For this review, take the finished solid that the model builds, in its own axes (mm). Give positions to 0.01 mm unless a question says otherwise; leave off trailing zeros. Write each loop counter-clockwise with the first axis right and the second up, starting at its lowest first coordinate (ties: lowest second). Pieces come first, ordered by that corner, then holes. Notation, with made-up numbers: (18, 12) -> (74, 12) arc R19 cw to (74, 21) -> close; hole circle Ø4 at (33, 6). An arc over 180 degrees is marked (long way). Answer as CSV lines item,"result".
```python
from build123d import *

# Parameters (mm, degrees)
F1_DEPTH = 1.1557


with BuildPart() as f1:
    # F0 (on Front) → F1 (new body)
    with BuildSketch(Plane.XZ):
        with BuildLine():
            Line((0, 200), (0, 0))
            Line((0, 0), (80, 0))
            Line((80, 0), (80, 149.5))
            ThreePointArc((80, 149.5), (102.5, 172), (125, 149.5))
            Line((125, 149.5), (125, 0))
            Line((125, 0), (170, 0))
            Line((170, 0), (170, 149.5))
            ThreePointArc((170, 149.5), (192.5, 172), (215, 149.5))
            Line((215, 149.5), (215, 0))
            Line((215, 0), (318, 0))
            Line((318, 0), (318, 149.5))
            ThreePointArc((318, 149.5), (340.5, 172), (363, 149.5))
            Line((363, 149.5), (363, 0))
            Line((363, 0), (600, 0))
            Line((600, 0), (600, 200))
            Line((600, 200), (0, 200))
        make_face()
    extrude(amount=F1_DEPTH)


solid = f1.part
```
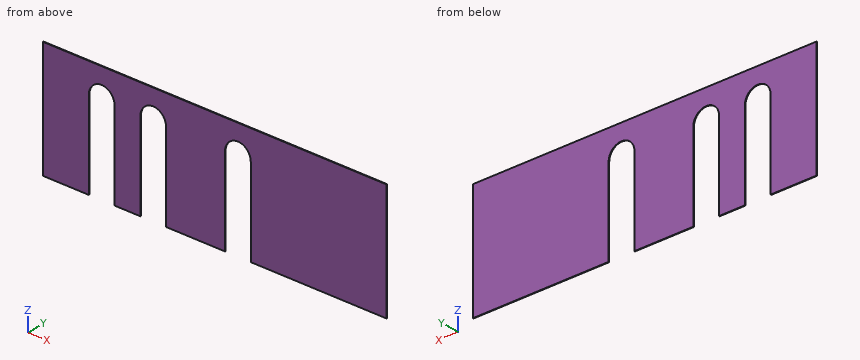
Q1. Add section A-A (z = 125). Write out the cut boundary in (x, y).
Answer block:
outline,"(0, -1.16) -> (80, -1.16) -> (80, 0) -> (0, 0) -> close; (125, -1.16) -> (170, -1.16) -> (170, 0) -> (125, 0) -> close; (215, -1.16) -> (318, -1.16) -> (318, 0) -> (215, 0) -> close; (363, -1.16) -> (600, -1.16) -> (600, 0) -> (363, 0) -> close"
Q2. Add section C-C (x = 340.5). Write out the cut boundary in (y, z), plus the area to 3 significant figures.
Answer block:
outline,"(-1.16, 172) -> (0, 172) -> (0, 200) -> (-1.16, 200) -> close"
area,"32.4 mm2"
Q3. To check wall thickness, follow probe 1 along X at (y, z) = (-0.85, 52.5); probe 2 along Z at (x, y) = (201.5, -0.8); probe 3 along Z at (x, y) = (348, -0.3). State the ranges of each line that lie inside material, in increasing order. Write a range as [from, to].
Answer block:
probe 1,"x = [0, 80], [125, 170], [215, 318], [363, 600]"
probe 2,"z = [170.12, 200]"
probe 3,"z = [170.71, 200]"
Q4. Add section B-B (y = -0.5). Write out the cut boundary in (x, z), plus the area to 3 significant figures.
Answer block:
outline,"(0, 0) -> (80, 0) -> (80, 149.5) arc R22.5 cw to (125, 149.5) -> (125, 0) -> (170, 0) -> (170, 149.5) arc R22.5 cw to (215, 149.5) -> (215, 0) -> (318, 0) -> (318, 149.5) arc R22.5 cw to (363, 149.5) -> (363, 0) -> (600, 0) -> (600, 200) -> (0, 200) -> close"
area,"97,400 mm2"
Q5. Add section D-D (z = 162.5). Write out the cut boundary in (x, y), plus the area to 3 significant figures.
Answer block:
outline,"(0, -1.16) -> (84.14, -1.16) -> (84.14, 0) -> (0, 0) -> close; (120.86, -1.16) -> (174.14, -1.16) -> (174.14, 0) -> (120.86, 0) -> close; (210.86, -1.16) -> (322.14, -1.16) -> (322.14, 0) -> (210.86, 0) -> close; (358.86, -1.16) -> (600, -1.16) -> (600, 0) -> (358.86, 0) -> close"
area,"566 mm2"
